Geometry check sheet. Reference: drawing and pictorial views, mm from the part's lowest x, y, z. Round coordinates to 2 decimals unless told otherwise and drop trailing zeros. Write each loop counter-clockwise with the first axis right and the second up, starting at its lowest first coordinate (ties: lowest second). Pieces come first, ordered by that corner, then holes. Notation, with made-up numbers: M -28.75,27 L 0.25,27 A22 cw 0.25,66 Z; hole C 23.25,-39.5 d7. An arc over 180 degrees is marked long. Answer in a Markdown table with one row per item.
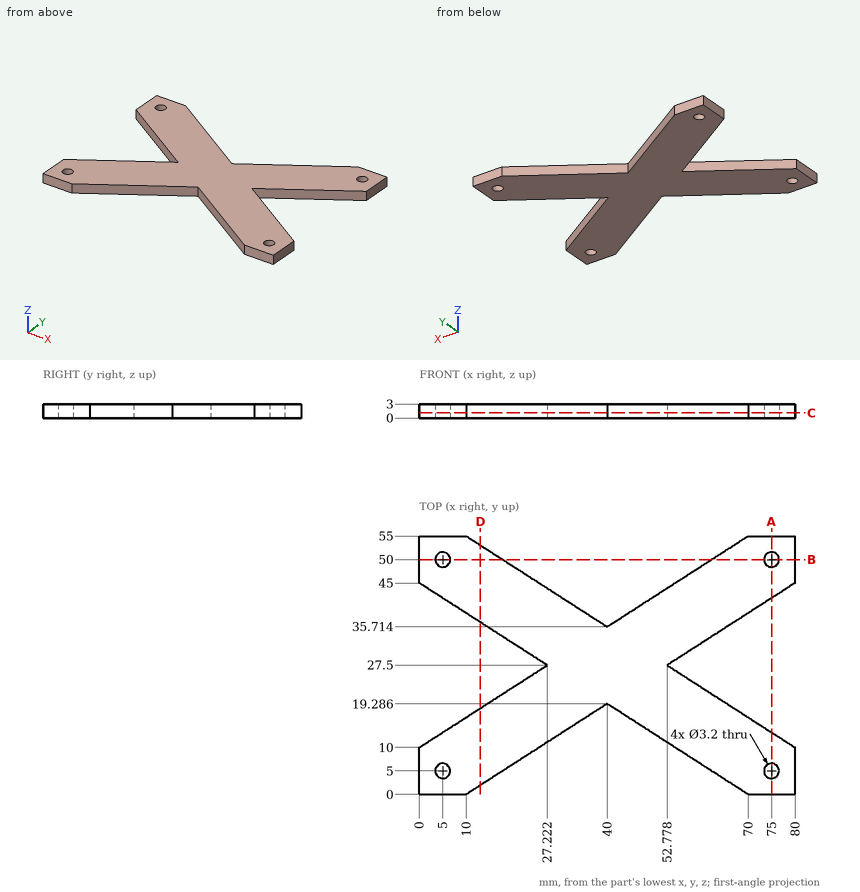
1. Section check C-C, the plane z = 1.1. Record the cut outline in (x, y), and give its area (3 significant figures).
Found:
| item | result |
|---|---|
| outline | M 0,0 L 10,0 L 40,19.29 L 70,0 L 80,0 L 80,10 L 52.78,27.5 L 80,45 L 80,55 L 70,55 L 40,35.71 L 10,55 L 0,55 L 0,45 L 27.22,27.5 L 0,10 Z; hole C 5,5 d3.2; hole C 5,50 d3.2; hole C 75,5 d3.2; hole C 75,50 d3.2 |
| area | 2,260 mm2 |
2. Go/stop test with a flat-tipped pin: pin 1 (3 mm diameter, centred on x = 5, y = 50, fed in from -Z). Record where the tip stops, or that it passes through.
Found:
| item | result |
|---|---|
| pin 1 | passes through |
3. Section check D-D, the plane x = 13. Record the cut outline in (y, z).
Found:
| item | result |
|---|---|
| outline | M 1.93,0 L 18.36,0 L 18.36,3 L 1.93,3 Z; M 36.64,0 L 53.07,0 L 53.07,3 L 36.64,3 Z |
4. Section check B-B, the plane y = 50. Record the cut outline in (x, z).
Found:
| item | result |
|---|---|
| outline | M 0,0 L 3.4,0 L 3.4,3 L 0,3 Z; M 6.6,0 L 17.78,0 L 17.78,3 L 6.6,3 Z; M 62.22,0 L 73.4,0 L 73.4,3 L 62.22,3 Z; M 76.6,0 L 80,0 L 80,3 L 76.6,3 Z |
5. Scan lines: L1, parallel to Y at x = 5, z = 1.55 (1 decimal); L2, parallel to Y at x = 76, z = 0.7; L3, parallel to Y at x = 16, z = 1.7 (1 decimal). Record each from-to range of solid material in increasing order.
Found:
| item | result |
|---|---|
| L1 | y = 0 to 3.4, 6.6 to 13.2, 41.8 to 48.4, 51.6 to 55 |
| L2 | y = 0 to 3.75, 6.25 to 12.57, 42.43 to 48.75, 51.25 to 55 |
| L3 | y = 3.9 to 20.3, 34.7 to 51.1 |
6. Section check A-A, the plane x = 75. Record the cut outline in (y, z).
Found:
| item | result |
|---|---|
| outline | M 0,0 L 3.4,0 L 3.4,3 L 0,3 Z; M 6.6,0 L 13.21,0 L 13.21,3 L 6.6,3 Z; M 41.79,0 L 48.4,0 L 48.4,3 L 41.79,3 Z; M 51.6,0 L 55,0 L 55,3 L 51.6,3 Z |
